```python
from build123d import *

# Parameters (mm, degrees)
SKETCH1_W           = 105
SKETCH1_H           = 55
BOSS_EXTRUDE1_DEPTH = 10
SKETCH2_W           = 61
SKETCH2_H           = 31
CUT_EXTRUDE1_DEPTH  = 11
SKETCH4_R           = 3.125
SKETCH4_W           = 2.5
SKETCH4_H           = 6.35
CUT_EXTRUDE3_DEPTH  = 11
BOSS_EXTRUDE2_DEPTH = 10
SKETCH6_R           = 3.075
CUT_EXTRUDE4_DEPTH  = 11.0000001
FILLET1_R           = 4
FILLET2_R           = 0.5


with BuildPart() as part:
    # Sketch1 → Boss-Extrude1 (new body)
    with BuildSketch(Plane(origin=(0, 0, 0), x_dir=(1, 0, 0), z_dir=(0, 1, 0))):
        Rectangle(SKETCH1_W, SKETCH1_H)
    extrude(amount=BOSS_EXTRUDE1_DEPTH)

    # Sketch2 → Cut-Extrude1 (cut, through all)
    with BuildSketch(Plane(origin=(0, 10, 0), x_dir=(1, 0, 0), z_dir=(0, 1, 0))):
        with Locations((0, 3)):
            Rectangle(SKETCH2_W, SKETCH2_H)
    extrude(amount=-CUT_EXTRUDE1_DEPTH, mode=Mode.SUBTRACT)

    # Sketch4 → Cut-Extrude3 (cut, through all)
    with BuildSketch(Plane(origin=(0, 10, 0), x_dir=(1, 0, 0), z_dir=(0, 1, 0))):
        with Locations((-46.5, 3.5)):
            Circle(SKETCH4_R)
        with Locations((-34.5, 3.5)):
            Rectangle(SKETCH4_W, SKETCH4_H)
    cut_extrude3 = extrude(amount=-CUT_EXTRUDE3_DEPTH, mode=Mode.SUBTRACT)

    # Sketch5 → Boss-Extrude2 (add)
    with BuildSketch(Plane(origin=(0, 0, 0), x_dir=(1, 0, 0), z_dir=(0, 1, 0))):
        with BuildLine():
            Line((0, -27.5), (-52.5, -19.039128985))
            Line((-52.5, -19.039128985), (-60.28224578, -53.259137237))
            add(Edge.make_bspline(
                [(0, -27.5), (-47.690720084, -27.5), (-60.28224578, -53.259137237)],
                knots=[4.71238898, 4.71238898, 4.71238898, 6.015992757, 6.015992757, 6.015992757], degree=2, weights=[1, 0.794992028, 1]))
        make_face()
    boss_extrude2 = extrude(amount=BOSS_EXTRUDE2_DEPTH)

    # Sketch6 → Cut-Extrude4 (cut, through all)
    with BuildSketch(Plane(origin=(0, 10, 0), x_dir=(1, 0, 0), z_dir=(0, 1, 0))):
        with Locations((-44.108495475, 18.541732167)):
            Circle(SKETCH6_R)
    cut_extrude4 = extrude(amount=-CUT_EXTRUDE4_DEPTH, mode=Mode.SUBTRACT)

    # Mirror1: Cut-Extrude3, Boss-Extrude2, Cut-Extrude4 across plane
    add(cut_extrude3.mirror(Plane(origin=(0, 0, 0), x_dir=(0, 0, 1), z_dir=(1, 0, 0))), mode=Mode.SUBTRACT)
    add(boss_extrude2.mirror(Plane(origin=(0, 0, 0), x_dir=(0, 0, 1), z_dir=(1, 0, 0))))
    add(cut_extrude4.mirror(Plane(origin=(0, 0, 0), x_dir=(0, 0, 1), z_dir=(1, 0, 0))), mode=Mode.SUBTRACT)

    # Fillet1
    fillet1_edges = [part.edges().sort_by_distance(p)[0] for p in [
        (-52.5, 5, 19.039128985),
        (-52.5, 5, -27.5),
        (52.5, 5, -27.5),
        (52.5, 5, 19.039128985),
    ]]
    fillet(fillet1_edges, radius=FILLET1_R)

    # Fillet2
    fillet2_edges = [part.edges().sort_by_distance(p)[0] for p in [
        (60.28224578, 5, 53.259137237),
        (-60.28224578, 5, 53.259137237),
    ]]
    fillet(fillet2_edges, radius=FILLET2_R)


solid = part.part
```
Here's how the part is built. I have some questions about the finished solid (model axes, mm). A direction names the side the tool comes from. Coordinates: 2 decimals unless noted, no trailing zeros. Order: outer loops, then holes, each group sorted by start corner. A loop starts at its lowest first (then second) coordinate and runs counter-clockwise, first axis right, second up.
1) We'd pull the mould along Z, two halves only. Please class faces 3 (the face through (-35.75, 5, -3)), 4 (the face through (-52.5, 5, -2)), 5 (the face through (-30.5, 5, -3)), 6 (the face through (-51.359, 5.07, -26.297)): +Z half, -Z half, draft (parallel to the pull), parting line (faces both ways), or undercut.
2) I need wall thicknesses on line 1 (X direction, y = 6.5, z = -3.5) (3 decimals); line 2 (X direction, y = 2.5, z = 6); line 3 (Z direction, x = 46.5, y = 5) (3 decimals). Which ranges of each line are inside material? Lowest first, please.
3) Imagine slicing it at A-A on z = -3.5. List the corners of the cut face in (x, y) for me (3 decimals).
4) Imagine slicing it at B-B on y = 1.25. State how many separate pieces and enclosed holes the cut face has, and give its area (3 significant figures).
5) Which directions (+Z, -Z, +X, -X, +Y, -Y) give clear straight access to the entire face, cutting with the end or side of a thin tool? Please do faces 1 (the face through (-33.25, 5, -3)), 2 (the face through (-1, 5, -27.5)).
6) Will these pins go through, and if not, where does the flat tip stop? pin 1 (1 mm diameter, centred on y = 7.5, z = 31, fed in from -X); pin 2 (5 mm diameter, centred on y = 6.5, z = -5, fed in from -X); pin 3 (3 mm diameter, centred on x = 12.5, y = 2.5, fed in from +Z); pin 4 (7 mm diameter, centred on x = 46.5, z = -3.5, fed in from +Y).
Response values:
1. face 3: undercut
1. face 4: draft
1. face 5: undercut
1. face 6: -Z half
2. line 1: x = -52.5 to -49.625, -43.375 to -35.75, -33.25 to -30.5, 30.5 to 33.25, 35.75 to 43.375, 49.625 to 52.5
2. line 2: x = -52.5 to -30.5, 30.5 to 52.5
2. line 3: z = -27.5 to -20.475, -16.609 to -6.625, -0.375 to 39.114
3. outline: (-52.5, 0) - (-49.625, 0) - (-49.625, 10) - (-52.5, 10) - close; (-43.375, 0) - (-35.75, 0) - (-35.75, 10) - (-43.375, 10) - close; (-33.25, 0) - (-30.5, 0) - (-30.5, 10) - (-33.25, 10) - close; (30.5, 0) - (33.25, 0) - (33.25, 10) - (30.5, 10) - close; (35.75, 0) - (43.375, 0) - (43.375, 10) - (35.75, 10) - close; (49.625, 0) - (52.5, 0) - (52.5, 10) - (49.625, 10) - close
4. separate pieces: 1
4. enclosed holes: 7
4. area: 4,400 mm2
5. face 1: +Y, -Y
5. face 2: -Z, +X, -X, +Y, -Y
6. pin 1: stops at x = -55.33
6. pin 2: stops at x = -52.5
6. pin 3: stops at z = 28.39
6. pin 4: stops at y = 10
